from build123d import *

# Parameters (mm, degrees)
SKETCH_1_W          = 80
SKETCH_1_H          = 110
EXTRUDE_1_DEPTH     = 15
SKETCH_2_W          = 80
SKETCH_2_H          = 15
EXTRUDE_2_DEPTH     = 30
EXTRUDE_3_DEPTH     = 10
SKETCH_4_R          = 15
EXTRUDE_4_DEPTH     = 15
SKETCH_5_R          = 9
CUT_EXTRUDE_1_DEPTH = 75.330343737
SKETCH_6_R          = 6.5
CUT_EXTRUDE_2_DEPTH = 113.472218792
SKETCH_7_R          = 7.5
CUT_EXTRUDE_3_DEPTH = 126.39936204
SKETCH_8_W          = 16
SKETCH_8_H          = 7
CUT_EXTRUDE_4_DEPTH = 82.547532274


with BuildPart() as part:
    # Эскиз1 → Бобышка-Вытянуть1 (new body)
    with BuildSketch(Plane.XY):
        Rectangle(SKETCH_1_W, SKETCH_1_H)
    extrude(amount=EXTRUDE_1_DEPTH)

    # Эскиз2 → Бобышка-Вытянуть2 (add)
    with BuildSketch(Plane.XY.offset(15)):
        with Locations((0, 47.5)):
            Rectangle(SKETCH_2_W, SKETCH_2_H)
    extrude(amount=EXTRUDE_2_DEPTH)

    # Эскиз3 → Бобышка-Вытянуть3 (add)
    with BuildSketch(Plane(origin=(40, 0, 0), x_dir=(0, 0, -1), z_dir=(1, 0, 0))):
        Polygon((-39, 40), (-15, -30), (-15, 40), align=None)
    extrude_3 = extrude(amount=-EXTRUDE_3_DEPTH)

    # Зеркальное отражение1: Бобышка-Вытянуть3 across plane
    add(extrude_3.mirror(Plane(origin=(0, 0, 0), x_dir=(0, 0, 1), z_dir=(1, 0, 0))))

    # Эскиз4 → Бобышка-Вытянуть4 (add)
    with BuildSketch(Plane.XY.offset(15)):
        with Locations(Location((0, 0, 0), (0, 0, 180))):
            Circle(SKETCH_4_R)
    extrude(amount=EXTRUDE_4_DEPTH)

    # Эскиз5 → Вырез-Вытянуть1 (cut, through all)
    with BuildSketch(Plane.XY.offset(30)):
        Circle(SKETCH_5_R)
    extrude(amount=-CUT_EXTRUDE_1_DEPTH, mode=Mode.SUBTRACT)

    # Эскиз6 → Вырез-Вытянуть2 (cut, through all)
    with BuildSketch(Plane.XZ.offset(-40)):
        with Locations((0, 30)):
            Circle(SKETCH_6_R)
    extrude(amount=-CUT_EXTRUDE_2_DEPTH, mode=Mode.SUBTRACT)

    # Эскиз7 → Вырез-Вытянуть3 (cut, through all)
    with BuildSketch(Plane.XZ.offset(55)):
        Circle(SKETCH_7_R)
    extrude(amount=-CUT_EXTRUDE_3_DEPTH, mode=Mode.SUBTRACT)

    # Эскиз8 → Вырез-Вытянуть4 (cut, through all)
    with BuildSketch(Plane.XY.offset(45)):
        with Locations((0, 51.5)):
            Rectangle(SKETCH_8_W, SKETCH_8_H)
    extrude(amount=-CUT_EXTRUDE_4_DEPTH, mode=Mode.SUBTRACT)


solid = part.part
Work out the finished part from the listing and answer in its coordinate system (mm). A direction names the side the tool comes from. Coordinates: 2 decimals unless noted, no trailing zeros. Loops run counter-clockwise (first coordinate to the right, second up) from the corner with the lowest first, then second, coordinate; pieces in that order, holes last. Notation, with made-up numbers: M 61.25,-7 L 71.25,-7 A26 cw 71.25,19 Z; hole C 42,37 d3. An arc over 180 degrees is marked long. Answer in a Markdown table with one row per item. Add a question column.
1. The mould has two halves that part along Y. Classify faces 1 (the flat face through (-1, 40, 23)), 2 (the flat face through (24, 55, 22)), 3 (the flat face through (-35, 5, 27)), 4 (the flat face through (-0.6, 47.6, 45)): pulls with the +Y half, pulls with the -Y half, needs draft (parallel to the pull), parting line crosses it, or undercut.
2. Find section D-D, the plane y = 0. Write down the section's boundary in (x, z).
3. Find section C-C, the plane x = 0. Write down the section's boundary in (y, z), then the cut area to 4 significant figures.
4. Flat-ended cylindrical pins translate along their axes: P1, Ø9, axis at x = -3, z = 28, coming from the -Y side; P2, Ø3, axis at y = -17.5, z = 30, coming from the +X side; P3, Ø15, axis at x = -5, y = 7.5, coming from the +Z side; P4, Ø2, axis at x = -14, y = 27.5, coming from the +Z side. Find the tip coordinate at first contact, or state that the pin passes through.
5. Consider L1, parallel to Y at x = 0, z = 18; L2, parallel to X at y = -12, z = 18; L3, parallel to Z at x = 0, y = 45.25. Determine where each line is inside the solid, lowest interval first.
6. Find section B-B, the plane z = 27. Write down the section's boundary in (x, y).
7. Find section A-A, the plane z = 21. Write down the section's boundary in (x, y).
8. A tool of negligible diameter and unlimited length cuts with its end or side. For faces 5 (the flat face through (8, 51, 23)), 6 (the flat face through (35, 5, 27)), 7 (the flat face through (30, 21, 22)), from which of +Z, -Z, +X, -X, +Y, -Y can it reach the whole face along a straight path? Write none if from no direction.
Reported:
| question | item | result |
|---|---|---|
| 1 | face 1 | undercut |
| 1 | face 2 | pulls with the +Y half |
| 1 | face 3 | pulls with the -Y half |
| 1 | face 4 | needs draft |
| 2 | outline | M -40,0 L -9,0 L -9,30 L -15,30 L -15,15 L -30,15 L -30,25.29 L -40,25.29 Z; M 9,0 L 40,0 L 40,25.29 L 30,25.29 L 30,15 L 15,15 L 15,30 L 9,30 Z |
| 3 | outline | M -55,7.5 L -9,7.5 L -9,30 L -15,30 L -15,15 L -55,15 Z; M 9,7.5 L 48,7.5 L 48,23.5 L 40,23.5 L 40,15 L 15,15 L 15,30 L 9,30 Z; M 40,36.5 L 48,36.5 L 48,45 L 40,45 Z |
| 3 | area | 953.5 mm^2 |
| 4 | P1 | stops at y = -15 |
| 4 | P2 | passes through |
| 4 | P3 | stops at z = 30 |
| 4 | P4 | stops at z = 15 |
| 5 | L1 | y = -15 to -9, 9 to 15, 40 to 48 |
| 5 | L2 | x = -40 to -30, -9 to 9, 30 to 40 |
| 5 | L3 | z = 7.5 to 23.5, 36.5 to 45 |
| 6 | outline | M -40,5 L -30,5 L -30,40 L -5.77,40 L -5.77,48 L -8,48 L -8,55 L -40,55 Z; C 0,0 d30; M 5.77,40 L 30,40 L 30,5 L 40,5 L 40,55 L 8,55 L 8,48 L 5.77,48 Z; hole C 0,0 d18 |
| 7 | outline | M -40,-12.5 L -30,-12.5 L -30,40 L 30,40 L 30,-12.5 L 40,-12.5 L 40,55 L 8,55 L 8,48 L -8,48 L -8,55 L -40,55 Z; C 0,0 d30; hole C 0,0 d18 |
| 8 | face 5 | +Z, -Z, +Y |
| 8 | face 6 | +Z, +X, -Y |
| 8 | face 7 | +Z, -Y |
